Here's how the part is built. I have some questions about the finished solid (model axes, mm). A direction names the side the tool comes from. Give positions to 0.01 mm unless a question says otherwise; leave off trailing zeros. Order: outer loops, then holes, each group sorted by start corner. A loop starts at its lowest first (then second) coordinate and runs counter-clockwise, first axis right, second up.
from build123d import *

# Parameters (mm, degrees)
F1_DEPTH = 63.5
F0_W     = 8.383435
F0_H     = 19.05
F2_DEPTH = 25.4
F3_DEPTH = 7.9375
F5_R     = 6.35


with BuildPart() as f1:
    # F0 (on Front) → F1 (new body, symmetric)
    with BuildSketch(Plane.XZ):
        Polygon((-41.275, 9.525), (-41.275, -9.525), (41.275, -9.525), (41.275, 9.525), (22.225, 9.525), align=None)
    extrude(amount=F1_DEPTH, both=True)

    # F0 (on Front) → F2 (join, symmetric)
    with BuildSketch(Plane.XZ):
        with BuildLine():
            Line((22.225, 9.525), (41.275, 9.525))
            Line((41.275, 9.525), (41.275, 26.141635))
            ThreePointArc((41.275, 26.141635), (44.340935, 35.519453), (52.354492, 41.275))
            Line((52.354492, 41.275), (60.325, 41.275))
            Line((60.325, 41.275), (60.325, 60.325))
            Line((60.325, 60.325), (49.990866, 60.325))
            ThreePointArc((49.990866, 60.325), (30.041068, 48.161205), (22.225, 26.141635))
            Line((22.225, 26.141635), (22.225, 9.525))
        make_face()
        with Locations((64.516717, 50.8)):
            Rectangle(F0_W, F0_H)
    extrude(amount=F2_DEPTH, both=True)

    # F0 (on Front) → F3 (join, symmetric)
    with BuildSketch(Plane.XZ):
        with BuildLine():
            add(Edge.make_bspline(
                [(-41.275, 9.525), (-40.494805, 46.327003), (24.913717, 63.209177), (60.325, 60.325)],
                knots=[0, 0, 0, 0, 113.592253, 113.592253, 113.592253, 113.592253], degree=3))
            Line((-41.275, 9.525), (22.225, 9.525))
            Line((22.225, 9.525), (22.225, 26.141635))
            ThreePointArc((22.225, 26.141635), (30.041068, 48.161205), (49.990866, 60.325))
            Line((49.990866, 60.325), (60.325, 60.325))
        make_face()
    extrude(amount=F3_DEPTH, both=True)

    # F0 (on Front) → F4 (revolve)
    with BuildSketch(Plane.XZ):
        Polygon((68.708435, 66.675), (68.708435, 60.325), (68.708435, 41.275), (68.708435, 38.1), (111.125, 38.1), (111.125, 66.675), align=None)
    revolve(axis=Axis((68.708435, 0, 52.3875), (0, 0, -1)))

    # F5
    f5_edges = [f1.edges().sort_by_distance(p)[0] for p in [
        (-41.275, -63.5, 0),
        (41.275, -63.5, 0),
        (-41.275, 63.5, 0),
        (41.275, 63.5, 0),
    ]]
    fillet(f5_edges, radius=F5_R)


solid = f1.part
Q1. If we section it at B-B on y = 16.5: List the corners of the cut face in (x, z) for me (3 decimals).
Filled sheet:
outline: (-41.275, -9.525) - (41.275, -9.525) - (41.275, 26.142) arc R15.875 cw to (46.709, 38.1) - (107.784, 38.1) - (107.784, 66.675) - (29.633, 66.675) - (29.633, 47.649) arc R34.925 ccw to (22.225, 26.142) - (22.225, 9.525) - (-41.275, 9.525) - close
Q2. Thinking about a two-plate mould opening in Z: for faces 4 (the face through (-1, -1, -9.525)), 5 (the face through (32, -25.4, 27)), 6 (the face through (32, 25.4, 27)), 7 (the face through (39.464, -61.59, 0.133)), which applies, released by +Z, released by -Z, zero draft, split by the parting line, or undercut?
Filled sheet:
face 4: released by -Z
face 5: undercut
face 6: undercut
face 7: zero draft
Q3. For faces 1 (the face through (22.225, 17, 18)), 2 (the face through (41.275, -1, 4)), 3 (the face through (109.166, -12.741, 52.588)), which set-ups out of +Z, -Z, +X, -X, +Y, -Y let a thin tool reach every point of the face, with its end or its side?
Filled sheet:
face 1: +Z, -X, +Y
face 2: -Z, +X, +Y, -Y
face 3: +Z
Q4. I'm going to push flat-ended pins straight in: P1, Ø12, axis at y = 37, z = 48.5, coming from the -X side; P2, Ø23, axis at x = 59, y = -13, coming from the -Z side; P3, Ø3, axis at x = 67, z = 53.5, coming from the +Y side. Where does each tip first touch, or does it pass through?
Filled sheet:
P1: stops at x = 39.76
P2: stops at z = 38.1
P3: stops at y = 42.42
Q5. If we section it at D-D on y = -36: List the corners of the cut face in (x, z) for me (3 decimals), plus the area to 3 significant figures.
Filled sheet:
outline: (-41.275, -9.525) - (41.275, -9.525) - (41.275, 9.525) - (-41.275, 9.525) - close; (46.277, 38.1) - (91.14, 38.1) - (91.14, 66.675) - (46.277, 66.675) - close
area: 2,850 mm2
Q6. If we section it at C-C on x = 32: List the corners of the cut face in (y, z) for me (3 decimals).
Filled sheet:
outline: (-63.5, -9.525) - (63.5, -9.525) - (63.5, 9.525) - (25.4, 9.525) - (25.4, 50.375) - (21.252, 50.375) - (21.252, 66.675) - (-21.252, 66.675) - (-21.252, 50.375) - (-25.4, 50.375) - (-25.4, 9.525) - (-63.5, 9.525) - close
Q7. I need wall thicknesses on L1, parallel to X at y = 21, z = -6 (3 decimals); L2, parallel to Z at x = 70, y = -23 (3 decimals); L3, parallel to Z at x = -16, y = -26 (3 decimals). Which ranges of each line are inside material? Lowest first, please.
Filled sheet:
L1: x = -41.275 to 41.275
L2: z = 38.1 to 66.675
L3: z = -9.525 to 9.525
Q8. If we section it at A-A on y = 35: List the corners of the cut face in (x, z) for me (3 decimals).
Filled sheet:
outline: (-41.275, -9.525) - (41.275, -9.525) - (41.275, 9.525) - (-41.275, 9.525) - close; (44.747, 38.1) - (92.67, 38.1) - (92.67, 66.675) - (44.747, 66.675) - close
